Design review of the part built by this model. Coordinates are the model's own, in mm. Face numbers are marked on the shaded views. A direction names the side the tool comes from. Coordinates: 2 decimals unless noted, no trailing zeros. Write each loop counter-clockwise with the first axis right and the second up, starting at its lowest first coordinate (ties: lowest second). Pieces come first, ordered by that corner, then holes. Notation, with made-up numbers: M 66,20.25 L 109,20.25 A28 ccw 109,59.25 Z; hole C 36,19.5 d3. An arc over 180 degrees is marked long. One line per question, with ' | ' between items.
from build123d import *

# Parameters (mm, degrees)
F1_DEPTH = 203.2
F2_R     = 50.8
F3_DEPTH = 203.2
F4_R     = 44.45
F5_DEPTH = 203.2
F6_W     = 355.6
F6_H     = 355.6
F7_DEPTH = 6.35
F8_R     = 3.175
F9_DEPTH = 6.35


with BuildPart() as f1:
    # F0 (on Right) → F1 (new body)
    with BuildSketch(Plane.YZ):
        Polygon((-101.6, 152.4), (-101.6, 0), (101.6, 0), (101.6, 152.4), (25.4, 284.382272), (-25.4, 284.382272), align=None)
    extrude(amount=F1_DEPTH)

    # F2 (on face) → F3 (join)
    with BuildSketch(Plane(origin=(0, 142.191136, 82.094091), x_dir=(-1, 0, 0), z_dir=(0, 0.866025, 0.5))):
        with Locations((-101.6, 157.382272)):
            Circle(F2_R)
    extrude(amount=F3_DEPTH)

    # F4 (on face) → F5 (join)
    with BuildSketch(Plane(origin=(0, -142.191136, 82.094091), x_dir=(1, 0, 0), z_dir=(0, -0.866025, 0.5))):
        with Locations((101.6, 157.382272)):
            Circle(F4_R)
    extrude(amount=F5_DEPTH)

    # F6 (on face) → F7 (join)
    with BuildSketch(Plane(origin=(0, 0, 0), x_dir=(1, 0, 0), z_dir=(0, 0, -1))):
        with Locations((101.6, 0)):
            Rectangle(F6_W, F6_H)
    extrude(amount=F7_DEPTH)

    # F8 (on face) → F9 (cut, through all)
    with BuildSketch(Plane(origin=(0, 0, -6.35), x_dir=(1, 0, 0), z_dir=(0, 0, -1))):
        with Locations((266.7, 165.1)):
            Circle(F8_R)
        with Locations((266.7, -165.1)):
            Circle(F8_R)
        with Locations((12.7, -165.1)):
            Circle(F8_R)
        with Locations((12.7, 165.1)):
            Circle(F8_R)
    extrude(amount=-F9_DEPTH, mode=Mode.SUBTRACT)


solid = f1.part
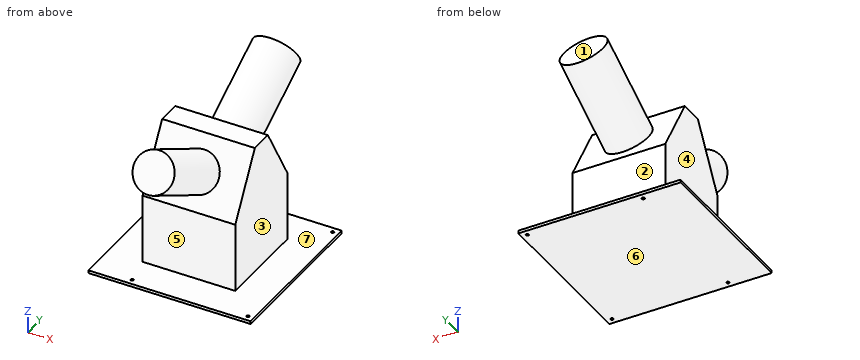
1. Insertion check: pin 1 Ø7 at (x, z) = (23.5, -4) entering from -Y; pin 2 Ø1 at (y, z) = (-198, 271.5) entering from -X; pin 3 Ø5 at (x, z) = (32.5, 221) entering from +Y; pin 4 Ø8.5 at (x, y) = (266.7, -165.1) entering from -Z. Each pin has a flat end and moves straight along its axis. Give the tip position at first contact, or say it passes through.
Answer sheet:
pin 1: y = -177.8 | pin 2: x = 62.29 | pin 3: y = 63.44 | pin 4: z = -6.35
2. To check wall thickness, follow line 1 along Y through (x, z) = (12.7, -4.5) (3 decimals); line 2 along X through (y, z) = (-165, -1); line 3 along Y through (x, z) = (12, -1). State the ranges of each line that lie inside material, in increasing order. Write a range as [from, to].
Answer sheet:
line 1: [-177.8, -168.275], [-161.925, 161.925], [168.275, 177.8] | line 2: [-76.2, 9.53], [15.87, 263.53], [269.87, 279.4] | line 3: [-177.8, -168.2], [-162, 162], [168.2, 177.8]
3. Draft analysis for pull direction Z (two halves, no side actions). For the marked faces 1, 2 and 3, state which applies: pulls with the +Z half, pulls with the -Z half, needs draft (parallel to the pull), parting line crosses it, or undercut.
Answer sheet:
face 1: pulls with the +Z half | face 2: undercut | face 3: needs draft
4. Take a section at C-C (x = -52.5). Write out the cut boundary in (y, z).
Answer sheet:
outline: M -177.8,-6.35 L 177.8,-6.35 L 177.8,0 L -177.8,0 Z
5. Take a section at A-A (x = 73). Write out the cut boundary in (y, z), then the cut area to 3 significant figures.
Answer sheet:
outline: M -256.49,290.52 L -80.51,188.92 L -101.6,152.4 L -101.6,0 L -177.8,0 L -177.8,-6.35 L 177.8,-6.35 L 177.8,0 L 101.6,0 L 101.6,152.4 L 84.49,182.03 L 260.47,283.63 L 218.48,356.35 L 42.51,254.75 L 25.4,284.38 L -25.4,284.38 L -46.49,247.86 L -222.46,349.46 Z | area: 80,900 mm^2
6. Tool access review of the marked faces 4, 5, 6 and 7: name each direction out of +Z, -Z, +X, -X, +Y, -Y from which nothing blocks a thin tool from reaching the whole face with its end or side.
Answer sheet:
face 4: +Z, -X, +Y, -Y | face 5: +X, -X, -Y | face 6: -Z, +X, -X, +Y, -Y | face 7: none
7. Take a section at B-B (z = 119). Write out the cut boundary in (x, y).
Answer sheet:
outline: M 0,-101.6 L 203.2,-101.6 L 203.2,101.6 L 0,101.6 Z
